Autodesk Inventor part; units mm, degrees
ref_plane "YZ Plane" through (0, 0, 0) normal (1, 0, 0) x (0, 1, 0)
ref_plane "XZ Plane" through (0, 0, 0) normal (0, 1, 0) x (-1, 0, 0)
ref_plane "XY Plane" through (0, 0, 0) normal (0, 0, 1) x (1, 0, 0)
sketch "Sketch1" plane through (0, 0, 0) normal (0, 1, 0) x (-1, 0, 0)
  line L0 (-22.5, 17.5) -> (22.5, 17.5)
  line L1 (22.5, 17.5) -> (22.5, -17.5)
  line L2 (22.5, -17.5) -> (-22.5, -17.5)
  line L3 (-22.5, -17.5) -> (-22.5, 17.5)
  line L4 (-22.5, 17.5) -> (22.5, -17.5) construction
  line L5 (22.5, 17.5) -> (-22.5, -17.5) construction
  point P0 (0, 0)
  dimension "d0" = 45
  dimension "d1" = 35
extrude "Extrusion1" add sketch "Sketch1" along normal mid plane 10
sketch "Sketch2" plane through (0, 5, 0) normal (0, 1, 0) x (1, 0, 0)
  point P0 (0, 0)
  point P1 (0, 0)
hole "Hole1" at (0, 5, 0) direction (0, -1, 0) diameter 19 end through all
sketch "Sketch3" plane through (0, 5, 0) normal (0, 1, 0) x (1, 0, 0)
  circle A0 centre (0, 0) radius 12 construction
  point P0 (0, 12)
  point P1 (12, 0)
  point P2 (0, -12)
  point P3 (-12, 0)
  dimension "d11" = 24
hole "Hole2" at (0, 5, -12) at (12, 5, 0) at (0, 5, 12) at (-12, 5, 0) direction (0, -1, 0) diameter 2.459 end through all
chamfer "Chamfer1" distance 0.2 angle 45 4 edges at (0, 5, -13.2295) (12, 5, -1.2295) (-12, 5, -1.2295) (0, 5, 10.7705)
chamfer "Chamfer2" distance 0.5 angle 45 2 edges at (0, 5, -9.5) (0, -5, -9.5)
sketch "Sketch4" plane through (-22.5, -5, 17.5) normal (0, 0, 1) x (1, 0, 0)
  line L0 (45, 0) -> (0, 0)
  line L1 (45, 0) -> (45, 10)
  line L2 (0, 10) -> (45, 10)
  line L3 (0, 0) -> (0, 10)
  point P0 (22.5, 5)
extrude "1" add sketch "Sketch4" along normal blind 15
sketch "Sketch7" plane through (-22.5, -5, 32.5) normal (0, 0, 1) x (1, 0, 0)
  line L0 (45, 10) -> (0, 10) construction
  line L1 (0, 10) -> (0, 0) construction
  line L2 (0, 0) -> (45, 0) construction
  line L3 (45, 0) -> (45, 10) construction
  line L4 (4, 10) -> (4, 22.65)
  line L5 (0, 10) -> (4, 10)
  line L6 (4, 22.65) -> (-36, 22.65)
  line L7 (6.5, 15) -> (6.5, 10) construction
  line L8 (0.5, 27.65) -> (0.5, 22.65) construction
  line L9 (-36, 12.65) -> (-36, 22.65)
  line L10 (-36, 12.65) -> (0, 12.65)
  line L11 (0, 12.65) -> (0, 10)
  point P0 (22.5, 5)
  dimension "d46" = 12.65
  dimension "d47" = 45
  dimension "d49" = 40
  dimension "d75" = 10
extrude "2" add sketch "Sketch7" against normal up to surface (50 mm away)
sketch "Sketch8" plane through (-58.5, 17.65, 32.5) normal (0, 1, 0) x (1, 0, 0)
  circle A0 centre (20.5, 32.5) radius 16
  circle A1 centre (32.5, 32.5) radius 3
  circle A2 centre (20.5, 20.5) radius 3
  circle A3 centre (8.5, 32.5) radius 3
  circle A4 centre (20.5, 44.5) radius 3
  circle A5 centre (20.5, 32.5) radius 6
  point P0 (58.5, 32.5)
hole "Hole4" at (-38, 17.65, 0) direction (0, -1, 0) diameter 19 end through all
hole "Hole5" at (-38, 17.65, -12) at (-26, 17.65, 0) at (-38, 17.65, 12) at (-50, 17.65, 0) direction (0, -1, 0) diameter 2.459 end through all
chamfer "Chamfer4" distance 0.2 angle 45 4 edges at (-38, 17.65, -13.2295) (-26, 17.65, -1.2295) (-50, 17.65, -1.2295) (-38, 17.65, 10.7705)
chamfer "Chamfer5" distance 0.5 angle 45 2 edges at (-38, 17.65, -9.5) (-38, 7.65, -9.5)
sketch "Sketch9" plane through (-22.5, -5, 32.5) normal (0, 0, 1) x (1, 0, 0)
  line L0 (-36, 22.65) -> (-36, 12.65) construction
  line L1 (0, 0) -> (45, 0) construction
  line L2 (-36, 22.65) -> (45, 22.65) construction
  line L3 (45, 22.65) -> (45, 0) construction
  line L4 (45, 0) -> (-36, 0) construction
  line L5 (-36, 0) -> (-36, 22.65) construction
  line L6 (-36, 22.65) -> (45, 0) construction
  line L7 (45, 22.65) -> (-36, 0) construction
  line L8 (45, -23.675) -> (-36, -23.675)
  line L9 (-36, -23.675) -> (-36, 46.325)
  line L10 (-36, 46.325) -> (45, 46.325)
  line L11 (45, 46.325) -> (45, -23.675)
  line L12 (45, -23.675) -> (-36, 46.325) construction
  line L13 (-36, -23.675) -> (45, 46.325) construction
  point P0 (22.5, 5)
  point P1 (4.5, 11.325)
  dimension "d76" = 81
  dimension "d77" = 70
extrude "Extrusion5" add sketch "Sketch9" along normal blind 15
sketch "Sketch11" plane through (-58.5, -28.675, 32.5) normal (0, -1, 0) x (1, 0, 0)
  line L0 (0, 0) -> (81, 0)
  line L1 (81, 0) -> (81, 15)
  line L2 (0, 15) -> (81, 15)
  line L3 (0, 0) -> (0, 15)
  point P0 (58.5, -32.5)
extrude "Extrusion6" add sketch "Sketch11" along normal blind 50
sketch "Sketch10" plane through (-22.5, -5, 47.5) normal (0, 0, 1) x (1, 0, 0)
  line L0 (45, 46.325) -> (-36, 46.325) construction
  line L1 (-36, 46.325) -> (-36, -73.675) construction
  line L2 (45, 46.325) -> (45, -73.675) construction
  line L3 (-36, 46.325) -> (-36, -23.675) construction
  line L4 (-20.5, -13.675) -> (29.5, -13.675) construction
  line L5 (29.5, -13.675) -> (29.5, 36.325) construction
  line L6 (29.5, 36.325) -> (-20.5, 36.325) construction
  line L7 (-20.5, 36.325) -> (-20.5, -13.675) construction
  line L8 (-20.5, -13.675) -> (29.5, 36.325) construction
  line L9 (29.5, -13.675) -> (-20.5, 36.325) construction
  line L10 (45, -73.675) -> (-36, -73.675)
  point P0 (4.5, 11.325)
  point P1 (-20.5, -63.675)
  point P2 (29.5, -63.675)
  dimension "d80" = 50
  dimension "d81" = 50
  dimension "d91" = 40.5
  dimension "d92" = 35
  dimension "d93" = 50
hole "Hole6" at (-43, 31.325, 47.5) at (7, 31.325, 47.5) at (7, -18.675, 47.5) at (-43, -18.675, 47.5) at (7, -68.675, 47.5) at (-43, -68.675, 47.5) direction (0, 0, -1) diameter 5.3 end through all
fillet "Fillet2" radius 8 4 edges at (0, -5, 32.5) (-40.5, 7.65, 32.5) (-38.5, 17.65, 32.5) (2, 5, 32.5)
fillet "Fillet3" radius 2 4 edges at (-18.5, 7.3431, 30.1569) (-18.5, 15.325, 32.5) (-18.5, 5, 3.5) (-22.5, 7.65, 3.5)
chamfer "Chamfer6" distance 0.2 angle 45 4 edges at (-43, -16.025, 32.5) (7, -16.025, 32.5) (-43, 33.975, 32.5) (7, 33.975, 32.5)
properties part number "KN-00-02-05" material "X5CrNi18-10"
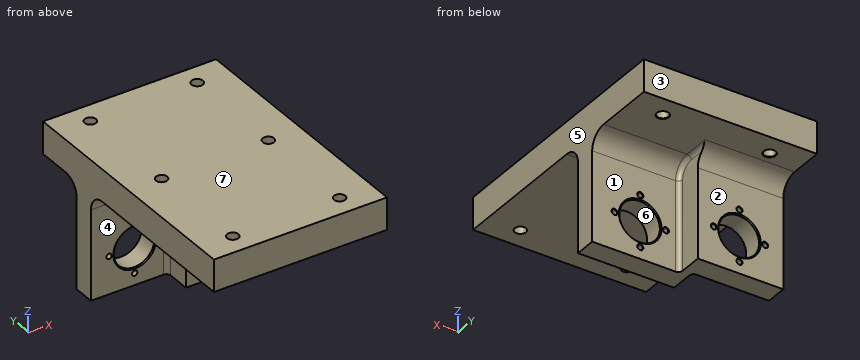
The listing builds one solid part. Answer for the finished solid, in the listing's coordinates (mm). Face numbers are marked on the shaded views. A direction names the side the tool comes from. Give positions to 0.01 mm unless a question says otherwise; leave off trailing zeros. Write each loop counter-clockwise with the first axis right and the second up, starting at its lowest first coordinate (ties: lowest second). Pieces come first, ordered by that corner, then holes. Notation, with made-up numbers: (-12.75, 67.5) -> (29.25, 67.5) arc R29 cw to (29.25, 88.5) -> close; hole circle Ø7 at (-17, -31). An arc over 180 degrees is marked (long way). Use a Markdown table: item, result.
(1) For the marked faces 1, 2, 3 and 4, determine the directions among +Z, -Z, +X, -X, +Y, -Y from which every point of the face is accessible in a straight line to the end or side of a thin tool.
Return value:
| item | result |
|---|---|
| face 1 | -Z, +X, +Y |
| face 2 | -Z, +X, -X, +Y |
| face 3 | +Z, -Z, +X, -X, +Y |
| face 4 | -Z, -X, -Y |
(2) Flat-ended cylindrical pins translate along their axes: P1, Ø4, axis at y = 0, z = 5, coming from the -X side; P2, Ø2, axis at x = 12, z = 0, coming from the -Y side; P3, Ø1, axis at x = -27.5, z = -8, coming from the -Y side; P4, Ø3, axis at x = 0, z = 12, coming from the -Y side. Find the tip coordinate at first contact, or state that the pin passes through.
Return value:
| item | result |
|---|---|
| P1 | x = -22.5 |
| P2 | through |
| P3 | y = 7.65 |
| P4 | y = -5 |
(3) Determine the mould class of the marked faces 5, 6 and 7 for opening direction X: released by +X, released by -X, zero draft, split by the parting line, or undercut.
Return value:
| item | result |
|---|---|
| face 5 | released by +X |
| face 6 | undercut |
| face 7 | zero draft |
(4) Section B-B, the plane y = -44.5 is taken. Determine the outline of the cut face in (x, z).
Return value:
| item | result |
|---|---|
| outline | (-58.5, 32.5) -> (22.5, 32.5) -> (22.5, 47.5) -> (-58.5, 47.5) -> close |
(5) Find the intervals of material crossed by probe 1 along Z at (x, y) = (-38, 11); probe 2 along X at (y, z) = (0.25, 0); probe 3 along X at (y, z) = (15.25, 0), in increasing order. Write a range as from..to.
Return value:
| item | result |
|---|---|
| probe 1 | -17.5..-13.23, -10.77..-9.5, 9.5..10.77, 13.23..47.5 |
| probe 2 | -22.5..-13.23, -10.77..-9.5, 9.5..10.77, 13.23..22.5 |
| probe 3 | -58.5..-51.23, -48.77..-47.5, -28.5..-27.23, -24.77..-18.5 |
(6) Section C-C, the plane z = 5 is taken. Give the number of separate pieces and of enclosed holes in the cut face, then the cut area to 3 significant figures.
Return value:
| item | result |
|---|---|
| separate pieces | 3 |
| enclosed holes | 0 |
| area | 538 mm2 |
(7) Section A-A, the plane z = 16.5 is taken. Determine the outline of the cut face in (x, y), then the cut area to 3 significant figures.
Return value:
| item | result |
|---|---|
| outline | (-58.5, 7.65) -> (-24.5, 7.65) arc R2 cw to (-22.5, 5.65) -> (-22.5, -5) -> (22.5, -5) -> (22.5, 5) -> (-16.5, 5) arc R2 cw to (-18.5, 7) -> (-18.5, 17.65) -> (-58.5, 17.65) -> close |
| area | 862 mm2 |
